Autodesk Inventor part; units mm, degrees
ref_plane "YZ Plane" through (0, 0, 0) normal (1, 0, 0) x (0, 1, 0)
ref_plane "XZ Plane" through (0, 0, 0) normal (0, 1, 0) x (-1, 0, 0)
ref_plane "XY Plane" through (0, 0, 0) normal (0, 0, 1) x (1, 0, 0)
sketch "Esquisse1" plane through (0, 0, 0) normal (0, 0, 1) x (1, 0, 0)
  line L0 (-6, 6) -> (-5, 6)
  line L1 (-5, 6) -> (-5, -5)
  line L2 (-5, -5) -> (-6, -5)
  line L3 (-6, -5) -> (-6, 6)
  line L4 (-5, 6) -> (5, 6)
  line L5 (5, 6) -> (5, 5)
  line L6 (5, 5) -> (-5, 5)
  line L7 (-5, 5) -> (-5, 6)
  point P0 (0, 0)
  dimension "d0" = 1
  dimension "d1" = 1
  dimension "d2" = 10
  dimension "d4" = 5
  dimension "d6" = 10
  dimension "d7" = 5
extrude "Extrusion1" add sketch "Esquisse1" along normal mid plane 10
sketch "Esquisse2" plane through (-5, 5, 5) normal (0, -1, 0) x (1, 0, 0)
  circle A0 centre (5, -5) radius 1.5
  dimension "d10" = 3
extrude "Extrusion2" cut sketch "Esquisse2" against normal through all
sketch "Esquisse3" plane through (-5, -5, 5) normal (1, 0, 0) x (0, 0, -1)
  circle A0 centre (5, 5) radius 1.5
  dimension "d13" = 3
extrude "Extrusion3" cut sketch "Esquisse3" against normal through all
properties part number "equerre"
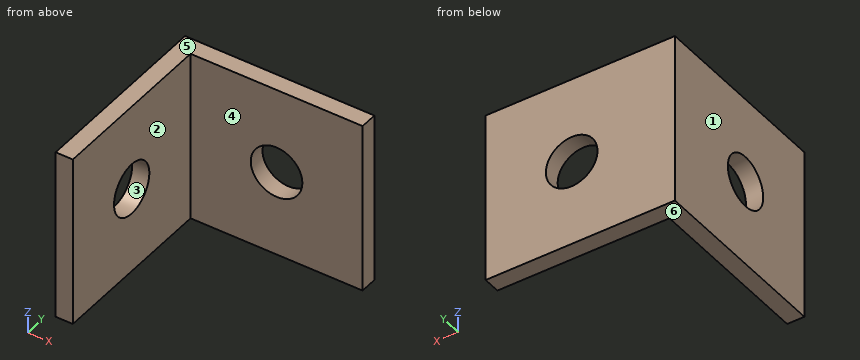
Geometry: final body of the model. Coordinates: model frame, mm. Face numbers are marked on the shaded views. A direction names the side the tool comes from. Give positions to 0.01 mm unless a question says otherwise; leave off trailing zeros. Write each loop counter-clockwise with the first axis right and the second up, starting at its lowest first coordinate (ties: lowest second). Pieces come first, ordered by that corner, then holes. Notation, with made-up numbers: (80.25, -38) -> (105.25, -38) arc R32 cw to (105.25, -10) -> close; hole circle Ø2 at (-39, 40.5). An arc over 180 degrees is marked (long way). Answer in a Markdown table with one row per item.
(1) Set-up query: the marked faces 1 and 2. Return all of +Z, -Z, +X, -X, +Y, -Y with unobstructed straight access to the full face (end or side cutting, diameter ignored); none if empty.
Answers below:
| item | result |
|---|---|
| face 1 | +Z, -Z, -X, +Y, -Y |
| face 2 | +Z, -Z, +X, -Y |
(2) Draft query along Z for the marked faces 3, 4, 5 and 6. Return one class per face: +Z half, -Z half, draft (parallel to the pull), parting line (faces both ways), or undercut.
Answers below:
| item | result |
|---|---|
| face 3 | undercut |
| face 4 | draft |
| face 5 | +Z half |
| face 6 | -Z half |
(3) Section query B-B on z = 0. Return loops of the section in (x, y).
Answers below:
| item | result |
|---|---|
| outline | (-6, -5) -> (-5, -5) -> (-5, -1.5) -> (-6, -1.5) -> close; (-6, 1.5) -> (-5, 1.5) -> (-5, 5) -> (-1.5, 5) -> (-1.5, 6) -> (-6, 6) -> close; (1.5, 5) -> (5, 5) -> (5, 6) -> (1.5, 6) -> close |
(4) Ray query, line 1 along Y through (x, z) = (-5.6, 0); line 2 along Y through (x, z) = (-0.25, -1.75); line 3 along X through (y, z) = (-4, 0.25). Return the intervals inside material, ascending. Write a range as [from, to].
Answers below:
| item | result |
|---|---|
| line 1 | [-5, -1.5], [1.5, 6] |
| line 2 | [5, 6] |
| line 3 | [-6, -5] |
(5) Section query D-D on z = 2.5. Return loops of the section in (x, y).
Answers below:
| item | result |
|---|---|
| outline | (-6, -5) -> (-5, -5) -> (-5, 5) -> (5, 5) -> (5, 6) -> (-6, 6) -> close |
(6) Section query A-A on y = 0. Return loops of the section in (x, z), then the cut area to 3 significant figures.
Answers below:
| item | result |
|---|---|
| outline | (-6, -5) -> (-5, -5) -> (-5, -1.5) -> (-6, -1.5) -> close; (-6, 1.5) -> (-5, 1.5) -> (-5, 5) -> (-6, 5) -> close |
| area | 7.00 mm^2 |
(7) Section query C-C on x = 0. Return loops of the section in (y, z).
Answers below:
| item | result |
|---|---|
| outline | (5, -5) -> (6, -5) -> (6, -1.5) -> (5, -1.5) -> close; (5, 1.5) -> (6, 1.5) -> (6, 5) -> (5, 5) -> close |
(8) Pin query (flat end, axial travel): pin 1 (1 mm diameter, centred on y = 2.5, z = 0.5, fed in from +X); pin 2 (4 mm diameter, centred on x = -2, z = -3.5, fed in from -Y). Return the tip coordinate at first contact, or that it passes through.
Answers below:
| item | result |
|---|---|
| pin 1 | x = -5 |
| pin 2 | y = 5 |
